Source: three-view drawing plus pictorial views. Frame: mm from the lowest corner of the part. A direction names the side the tool comes from. Round coordinates to 2 decimals unless told otherwise and drop trailing zeros. Loops run counter-clockwise (first coordinate to the right, second up) from the corner with the lowest first, then second, coordinate; pieces in that order, holes last. Notation, with made-up numbers: M -26.75,88 L -12.75,88 A9 ccw -12.75,99 Z; hole C -17.5,-32.5 d5. An arc over 180 degrees is marked long. Return JSON: item names as keys, results as strings. Group by question number.
1) Mould query, pull axis Y, two halves, no side actions, for the marked faces 4, 5, 6 and 7. Classes: +Y half, -Y half, draft (parallel to the pull), parting line (faces both ways), or undercut.
2) Section D-D (z = 6.25). Output: boundary loops of the cut face in (x, y) (1 decimal).
3) Contact query for flat-ended pins moving along their axis: P1, Ø4, axis at y = 11, z = 14, coming from the -X side; P2, Ø6, axis at x = 9.5, z = 12.5, coming from the +Y side; P3, Ø5, axis at y = 26.5, z = 21, coming from the -X side; P4, Ø5, axis at y = 17.5, z = 3.5, coming from the +X side. Output: stop coordinate, or through.
4) Section A-A (z = 12.7). Output: boundary loops of the cut face in (x, y) (1 decimal).
5) Section C-C (y = 29.5). Output: boundary loops of the cut face in (x, z).
6) Material intervals for line 1 (X direction, y = 1.2, z = 12.7); line 2 (Y direction, x = 62, z = 14.25) (1 decimal); line 3 (X direction, y = 9, z = 20) (1 decimal), sorted ascending. Write a range as from..to.
7) Access query for the marked faces 1, 2 and 3. Directions: +Z, -Z, +X, -X, +Y, -Y. A direction counts if a zero-diameter tool reaches every point of the face in a straight line with its end or side. Return the directions, or none.
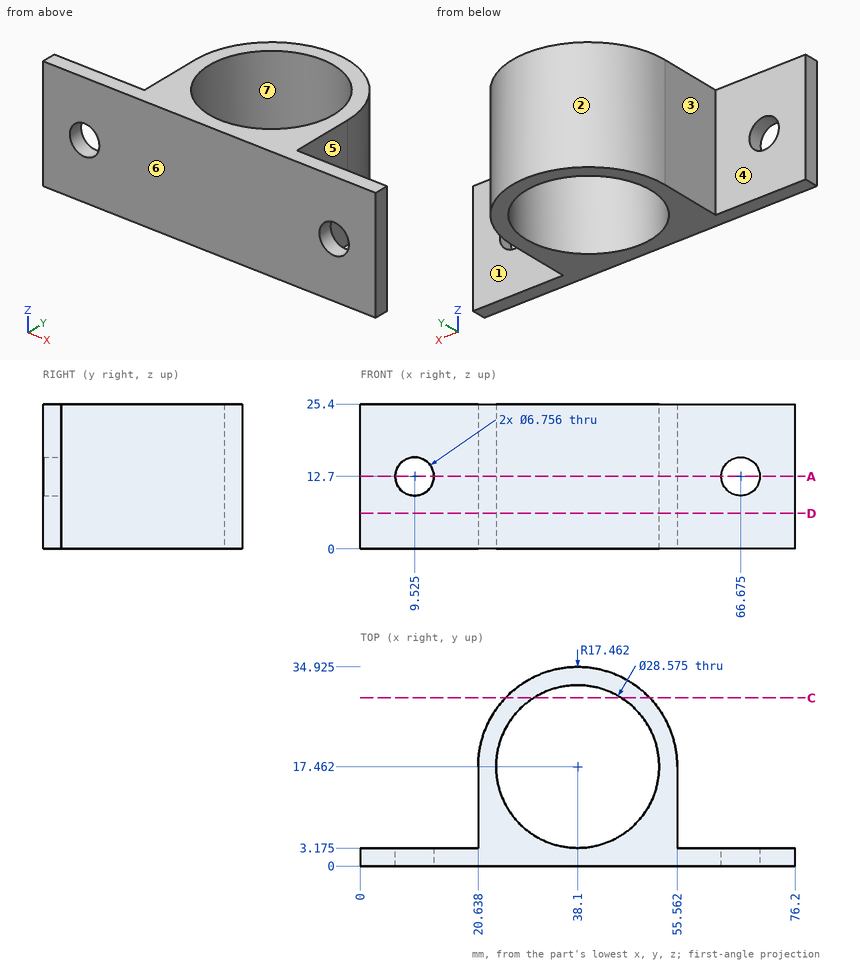
Returned:
{
 "1": {"face 4": "+Y half", "face 5": "draft", "face 6": "-Y half", "face 7": "undercut"},
 "2": {"outline": "M 0,0 L 76.2,0 L 76.2,3.2 L 55.6,3.2 L 55.6,17.5 A17.5 ccw 20.6,17.5 L 20.6,3.2 L 0,3.2 Z; hole C 38.1,17.5 d28.6"},
 "3": {"P1": "stops at x = 20.64", "P2": "passes through", "P3": "stops at x = 21.91", "P4": "stops at x = 55.56"},
 "4": {"outline": "M 0,0 L 6.1,0 L 6.1,3.2 L 0,3.2 Z; M 12.9,0 L 63.3,0 L 63.3,3.2 L 55.6,3.2 L 55.6,17.5 A17.5 ccw 20.6,17.5 L 20.6,3.2 L 12.9,3.2 Z; M 70.1,0 L 76.2,0 L 76.2,3.2 L 70.1,3.2 Z; hole C 38.1,17.5 d28.6"},
 "5": {"outline": "M 25.45,0 L 30.4,0 L 30.4,25.4 L 25.45,25.4 Z; M 45.8,0 L 50.75,0 L 50.75,25.4 L 45.8,25.4 Z"},
 "6": {"line 1": "x = 0..6.15, 12.9..63.3, 70.05..76.2", "line 2": "y = 0..3.2", "line 3": "x = 20.6..26.6, 49.6..55.6"},
 "7": {"face 1": "+Z, -Z, +X, +Y", "face 2": "+Z, -Z, +Y", "face 3": "+Z, -Z, -X, +Y"}
}
